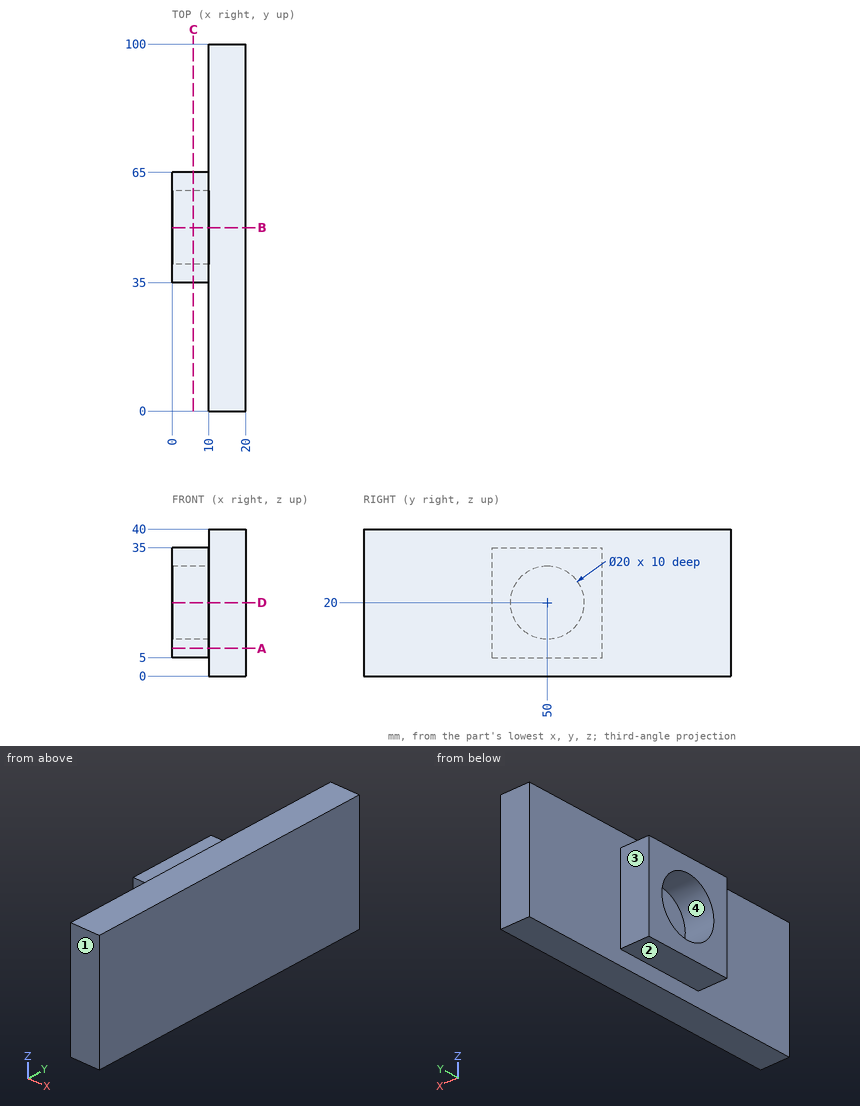
Could you check a few things on this drawing? It's one solid part, dimensions in mm from its lowest x, y, z. A direction names the side the tool comes from. Give positions to 0.01 mm unless a question says otherwise; leave off trailing zeros. Order: outer loops, then holes, each group sorted by start corner. A loop starts at its lowest first (then second) coordinate and runs counter-clockwise, first axis right, second up. Notation, with made-up numbers: (-1, 60.25) - (36, 60.25) arc R13 cw to (36, 85.25) - close; hole circle Ø6 at (14.25, 45.25). An arc over 180 degrees is marked (long way). Answer as a JSON object with one key per item and string values. Group by question number.
Item 1: For P1, Ø3, axis at x = 4, y = 47, coming from the +Z side; P2, Ø6, axis at y = 53, z = 19.5, coming from the -X side; P3, Ø5, axis at x = 6, z = 18, coming from the -Y side, each with a flat end and sliding along its axis, tell me the tip position at first contact or that it passes through.
Item 2: Please list where these lines run through material, in increasing order: probe 1 along Y at (x, z) = (5.5, 20); probe 2 along Y at (x, z) = (5.75, 33); probe 3 along X at (y, z) = (23, 33.5).
Item 3: If we section it at A-A on z = 7.5: Please give me the cut outline in (x, y), and give its area (3 significant figures).
Item 4: If we section it at C-C on x = 5.75: Please give me the cut outline in (y, z), and give its area (3 significant figures).
Item 5: If we section it at D-D on z = 20: Please give me the cut outline in (x, y), and give its area (3 significant figures).
Item 6: Which directions (+Z, -Z, +X, -X, +Y, -Y) give clear straight access to the entire face, cutting with the end or side of a thin tool? Please do the marked faces 1, 2, 3 and 4.
Item 7: If we section it at B-B on y = 50: Please give me the cut outline in (x, z).
Result set:
{
 "1": {"P1": "z = 35", "P2": "x = 10", "P3": "y = 35"},
 "2": {"probe 1": "35 to 40, 60 to 65", "probe 2": "35 to 65", "probe 3": "10 to 20"},
 "3": {"outline": "(0, 35) - (10, 35) - (10, 0) - (20, 0) - (20, 100) - (10, 100) - (10, 65) - (0, 65) - close", "area": "1,300 mm²"},
 "4": {"outline": "(35, 5) - (65, 5) - (65, 35) - (35, 35) - close; hole circle Ø20 at (50, 20)", "area": "586 mm²"},
 "5": {"outline": "(0, 35) - (10, 35) - (10, 0) - (20, 0) - (20, 100) - (10, 100) - (10, 65) - (0, 65) - (0, 60) - (10, 60) - (10, 40) - (0, 40) - close", "area": "1,100 mm²"},
 "6": {"face 1": "+Z, -Z, +X, -X, -Y", "face 2": "-Z, -X, +Y, -Y", "face 3": "+Z, -Z, -X, +Y", "face 4": "-X"},
 "7": {"outline": "(0, 5) - (10, 5) - (10, 0) - (20, 0) - (20, 40) - (10, 40) - (10, 35) - (0, 35) - (0, 30) - (10, 30) - (10, 10) - (0, 10) - close"}
}
